```python
from build123d import *

# Parameters (mm, degrees)
BOSS_EXTRUDE1_DEPTH      = 6
BOSS_EXTRUDE1_DEPTH_BACK = 3.525
FILLET1_R                = 1
CHAMFER1_SIZE            = 2
CHAMFER2_SIZE            = 0.5


with BuildPart() as part:
    # Sketch1 → Boss-Extrude1 (new body, two sides)
    with BuildSketch(Plane.XY) as boss_extrude1_sk:
        with BuildLine():
            Line((-10, 267.218866814), (-18.5, 258.718866814))
            ThreePointArc((-18.5, 258.718866814), (-20, 257.218866814), (-21.5, 258.718866814))
            Line((-21.5, 258.718866814), (-32.192388155, 269.41125497))
            Line((-32.192388155, 269.41125497), (-98.192388155, 269.41125497))
            Line((-98.192388155, 269.41125497), (-98.192388155, 239.41125497))
            Line((-98.192388155, 239.41125497), (-10, 239.41125497))
            Line((-10, 239.41125497), (-10, 267.218866814))
        make_face()
        with BuildLine():
            Line((-81.192388155, 262.16125497), (-91.192388155, 262.16125497))
            ThreePointArc((-91.192388155, 262.16125497), (-93.942388155, 259.41125497), (-91.192388155, 256.66125497))
            Line((-91.192388155, 256.66125497), (-81.192388155, 256.66125497))
            ThreePointArc((-81.192388155, 256.66125497), (-78.442388155, 259.41125497), (-81.192388155, 262.16125497))
        make_face(mode=Mode.SUBTRACT)
        with BuildLine():
            Line((-61.192388155, 262.16125497), (-71.192388155, 262.16125497))
            ThreePointArc((-71.192388155, 262.16125497), (-73.942388155, 259.41125497), (-71.192388155, 256.66125497))
            Line((-71.192388155, 256.66125497), (-61.192388155, 256.66125497))
            ThreePointArc((-61.192388155, 256.66125497), (-58.442388155, 259.41125497), (-61.192388155, 262.16125497))
        make_face(mode=Mode.SUBTRACT)
    extrude(amount=BOSS_EXTRUDE1_DEPTH)
    extrude(boss_extrude1_sk.sketch, amount=-BOSS_EXTRUDE1_DEPTH_BACK)

    # Fillet1
    fillet1_edges = [part.edges().sort_by_distance(p)[0] for p in [
        (-10, 267.218866814, 1.2375),
    ]]
    fillet(fillet1_edges, radius=FILLET1_R)

    # Chamfer1
    chamfer1_edges = [part.edges().sort_by_distance(p)[0] for p in [
        (-10, 239.41125497, 1.2375),
        (-98.192388155, 239.41125497, 1.2375),
    ]]
    chamfer(chamfer1_edges, length=CHAMFER1_SIZE)

    # Sketch3 → Cut-Revolve1 (revolve, cut)
    with BuildSketch(Plane(origin=(0, 0, 1.2375), x_dir=(-1, 0, 0), z_dir=(0, 0, -1))):
        Polygon((98.192388155, 250.91125497), (78.192388155, 250.91125497), (77.326362752, 249.41125497), (98.192388155, 249.41125497), align=None)
    revolve(axis=Axis((-98.192388155, 249.41125497, 1.2375), (-1, 0, 0)), mode=Mode.SUBTRACT)

    # Chamfer2
    chamfer2_edges = [part.edges().sort_by_distance(p)[0] for p in [
        (-98.192388155, 247.91125497, 1.2375),
    ]]
    chamfer(chamfer2_edges, length=CHAMFER2_SIZE)


solid = part.part
```
Build history of the part. All positions in model axes, mm. A direction names the side the tool comes from. Round coordinates to 2 decimals unless told otherwise and drop trailing zeros. Order: outer loops, then holes, each group sorted by start corner. A loop starts at its lowest first (then second) coordinate and runs counter-clockwise, first axis right, second up. Notation, with made-up numbers: (-28.75, 25.25) -> (15.25, 25.25) arc R32 cw to (15.25, 53.25) -> close; hole circle Ø4 at (26.25, 38.25). An arc over 180 degrees is marked (long way). Answer in a Markdown table with one row per item.
1) Pin check, flat tip, straight feed: P1, Ø2.5, axis at y = 249.41, z = 1.24, coming from the -X side. Stop position of the tip, or through.
Values:
| item | result |
|---|---|
| P1 | x = -78.05 |
2) Wall check: L1, parallel to X at y = 261, z = 1; L2, parallel to Y at x = -61, z = -1.5; L3, parallel to Y at x = -88.5, z = 0.5. Give the ranges that are in metal, low to high.
Values:
| item | result |
|---|---|
| L1 | -98.19 to -93.44, -78.95 to -73.44, -58.95 to -23.78, -16.22 to -10 |
| L2 | 239.41 to 256.67, 262.15 to 269.41 |
| L3 | 239.41 to 248.11, 250.72 to 256.66, 262.16 to 269.41 |
3) Mould opens along Z. For faces 1 (the flat face through (-55, 255, 6)), 2 (the cylindrical face through (-10.633, 265.735, 1.171)), 3 (the conical face through (-77.465, 249.172, 1.227)) say: released by +Z, released by -Z, zero draft, split by the parting line, or undercut.
Values:
| item | result |
|---|---|
| face 1 | released by +Z |
| face 2 | zero draft |
| face 3 | undercut |
4) Band-saw the part on A-A on z = 4. Give the cut face in (x, y).
Values:
| item | result |
|---|---|
| outline | (-98.19, 241.41) -> (-96.19, 239.41) -> (-12, 239.41) -> (-10, 241.41) -> (-10, 264.8) arc R1 ccw to (-11.71, 265.51) -> (-18.5, 258.72) arc R1.5 cw to (-21.5, 258.72) -> (-32.19, 269.41) -> (-98.19, 269.41) -> close; hole (-91.19, 256.66) -> (-81.19, 256.66) arc R2.75 ccw to (-81.19, 262.16) -> (-91.19, 262.16) arc R2.75 ccw to start; hole (-71.19, 256.66) -> (-61.19, 256.66) arc R2.75 ccw to (-61.19, 262.16) -> (-71.19, 262.16) arc R2.75 ccw to start |
5) Band-saw the part on B-B on x = -20. Give the cut face in (y, z) (3 decimals).
Values:
| item | result |
|---|---|
| outline | (239.411, -3.525) -> (257.219, -3.525) -> (257.219, 6) -> (239.411, 6) -> close |
6) Band-saw the part on C-C on y = 267. Give the cut face in (x, z) (3 decimals), and give its area (3 significant figures).
Values:
| item | result |
|---|---|
| outline | (-98.192, -3.525) -> (-29.781, -3.525) -> (-29.781, 6) -> (-98.192, 6) -> close |
| area | 652 mm2 |
7) Which spindle directions (+Z, -Z, +X, -X, +Y, -Y) get a long thin tool onto all of the face, cutting with end or side? Do faces 4 (the flat face through (-86, 262.161, 1)), 5 (the cylindrical face through (-87.806, 247.913, 1.172)), 6 (the flat face through (-10, 253, 1)), 7 (the flat face through (-26.77, 263.99, 1.3)). Say none if no direction does.
Values:
| item | result |
|---|---|
| face 4 | +Z, -Z |
| face 5 | -X |
| face 6 | +Z, -Z, +X, +Y, -Y |
| face 7 | +Z, -Z, +Y |
